For this review, take the finished solid that the model builds, in its own axes (mm). A direction names the side the tool comes from. Give positions to 0.01 mm unless a question says otherwise; leave off trailing zeros. Order: outer loops, then holes, each group sorted by start corner. A loop starts at its lowest first (then second) coordinate and runs counter-clockwise, first axis right, second up. Notation, with made-up numbers: (-11, -12) -> (-4, -12) arc R15 ccw to (-4, 11) -> close; hole circle Ø9 at (61.5, -27.75). An arc over 180 degrees is marked (long way). Use CSV: the item, a comma, the result in double quotes. Start each with the question number.
```python
from build123d import *

# Parameters (mm, degrees)
SKETCH_1_W               = 24
SKETCH_1_H               = 26
EXTRUDE_1_DEPTH          = 65
SKETCH_7_W               = 5
SKETCH_7_H               = 26
CUT_EXTRUDE_5_DEPTH      = 50
SKETCH_4_R               = 3
EXTRUDE_3_DEPTH          = 40
SKETCH_5_W               = 12.1
SKETCH_5_H               = 8
CUT_EXTRUDE_3_DEPTH      = 4
SKETCH_6_R               = 1
CUT_EXTRUDE_4_DEPTH      = 40
MIRROR_2_COPY_1_SKETCH_W = 5
MIRROR_2_COPY_1_SKETCH_H = 26
MIRROR_2_COPY_1_DEPTH    = 50
MIRROR_2_COPY_2_SKETCH_R = 3
MIRROR_2_COPY_2_DEPTH    = 40
MIRROR_2_COPY_3_SKETCH_W = 12.1
MIRROR_2_COPY_3_SKETCH_H = 8
MIRROR_2_COPY_3_DEPTH    = 4
MIRROR_2_COPY_4_SKETCH_R = 1
MIRROR_2_COPY_4_DEPTH    = 40
CUT_EXTRUDE_7_DEPTH      = 68.420693576
CUT_EXTRUDE_7_DEPTH_BACK = 68.420693576
CUT_EXTRUDE_8_REACH      = 83.979


with BuildPart() as part:
    # Эскиз1 → Бобышка-Вытянуть1 (new, symmetric)
    with BuildSketch(Plane.XY):
        with Locations((0, -0.287208972)):
            Rectangle(SKETCH_1_W, SKETCH_1_H)
    extrude(amount=EXTRUDE_1_DEPTH, both=True)

    # Эскиз7 → Вырез-Вытянуть5 (cut)
    with BuildSketch(Plane.XY.offset(65)):
        with Locations((-9.5, -0.287208972)):
            Rectangle(SKETCH_7_W, SKETCH_7_H)
    cut_extrude_5 = extrude(amount=-CUT_EXTRUDE_5_DEPTH, mode=Mode.SUBTRACT)

    # Эскиз4 → Бобышка-Вытянуть3 (add)
    with BuildSketch(Plane.XY.offset(65)):
        with BuildLine():
            ThreePointArc((-4, -10.287208972), (-4.878679656, -8.165888628), (-7, -7.287208972))
            Line((-7, -7.287208972), (-7, -13.287208972))
            ThreePointArc((-7, -13.287208972), (-4.878679656, -12.408529315), (-4, -10.287208972))
        make_face()
        with BuildLine():
            Line((-7, -13.287208972), (-7, -7.287208972))
            ThreePointArc((-7, -7.287208972), (-10, -10.287208972), (-7, -13.287208972))
        make_face()
        with Locations((-7, 9.712791028)):
            Circle(SKETCH_4_R)
    extrude_3 = extrude(amount=-EXTRUDE_3_DEPTH)

    # Эскиз5 → Вырез-Вытянуть3 (cut, symmetric)
    with BuildSketch(Plane.ZY.offset(7)):
        with Locations((45, -9.287208972)):
            Rectangle(SKETCH_5_W, SKETCH_5_H)
        with Locations((45, 8.712791028)):
            Rectangle(SKETCH_5_W, SKETCH_5_H)
    cut_extrude_3 = extrude(amount=CUT_EXTRUDE_3_DEPTH, both=True, mode=Mode.SUBTRACT)

    # Эскиз6 → Вырез-Вытянуть4 (cut)
    with BuildSketch(Plane.XY.offset(65)):
        with Locations((-7, 9.712791028)):
            Circle(SKETCH_6_R)
        with Locations((-7, -10.287208972)):
            Circle(SKETCH_6_R)
    cut_extrude_4 = extrude(amount=-CUT_EXTRUDE_4_DEPTH, mode=Mode.SUBTRACT)

    # Зеркальное отражение1: Вырез-Вытянуть5, Бобышка-Вытянуть3, Вырез-Вытянуть3, Вырез-Вытянуть4 across plane
    add(cut_extrude_5.mirror(Plane.XY), mode=Mode.SUBTRACT)
    add(extrude_3.mirror(Plane.XY))
    add(cut_extrude_3.mirror(Plane.XY), mode=Mode.SUBTRACT)
    add(cut_extrude_4.mirror(Plane.XY), mode=Mode.SUBTRACT)

    # Зеркальное отражение2: Вырез-Вытянуть5, Бобышка-Вытянуть3, Вырез-Вытянуть3, Вырез-Вытянуть4 across plane
    add(cut_extrude_5.mirror(Plane(origin=(0, 0, 0), x_dir=(0, 0, 1), z_dir=(1, 0, 0))), mode=Mode.SUBTRACT)
    add(extrude_3.mirror(Plane(origin=(0, 0, 0), x_dir=(0, 0, 1), z_dir=(1, 0, 0))))
    add(cut_extrude_3.mirror(Plane(origin=(0, 0, 0), x_dir=(0, 0, 1), z_dir=(1, 0, 0))), mode=Mode.SUBTRACT)
    add(cut_extrude_4.mirror(Plane(origin=(0, 0, 0), x_dir=(0, 0, 1), z_dir=(1, 0, 0))), mode=Mode.SUBTRACT)

    # Зеркальное отражение2 copy 1 sketch → Зеркальное отражение2 copy 1 (cut)
    with BuildSketch(Plane(origin=(0, 0, -65), x_dir=(-1, 0, 0), z_dir=(0, 0, -1))):
        with Locations((-9.5, -0.287208972)):
            Rectangle(MIRROR_2_COPY_1_SKETCH_W, MIRROR_2_COPY_1_SKETCH_H)
    extrude(amount=-MIRROR_2_COPY_1_DEPTH, mode=Mode.SUBTRACT)

    # Зеркальное отражение2 copy 2 sketch → Зеркальное отражение2 copy 2 (add)
    with BuildSketch(Plane(origin=(0, 0, -65), x_dir=(-1, 0, 0), z_dir=(0, 0, -1))):
        with BuildLine():
            ThreePointArc((-4, -10.287208972), (-4.878679656, -8.165888628), (-7, -7.287208972))
            Line((-7, -7.287208972), (-7, -13.287208972))
            ThreePointArc((-7, -13.287208972), (-4.878679656, -12.408529315), (-4, -10.287208972))
        make_face()
        with BuildLine():
            Line((-7, -13.287208972), (-7, -7.287208972))
            ThreePointArc((-7, -7.287208972), (-10, -10.287208972), (-7, -13.287208972))
        make_face()
        with Locations((-7, 9.712791028)):
            Circle(MIRROR_2_COPY_2_SKETCH_R)
    extrude(amount=-MIRROR_2_COPY_2_DEPTH)

    # Зеркальное отражение2 copy 3 sketch → Зеркальное отражение2 copy 3 (cut, symmetric)
    with BuildSketch(Plane(origin=(7, 0, 0), x_dir=(0, 0, -1), z_dir=(1, 0, 0))):
        with Locations((45, -9.287208972)):
            Rectangle(MIRROR_2_COPY_3_SKETCH_W, MIRROR_2_COPY_3_SKETCH_H)
        with Locations((45, 8.712791028)):
            Rectangle(MIRROR_2_COPY_3_SKETCH_W, MIRROR_2_COPY_3_SKETCH_H)
    extrude(amount=MIRROR_2_COPY_3_DEPTH, both=True, mode=Mode.SUBTRACT)

    # Зеркальное отражение2 copy 4 sketch → Зеркальное отражение2 copy 4 (cut)
    with BuildSketch(Plane(origin=(0, 0, -65), x_dir=(-1, 0, 0), z_dir=(0, 0, -1))):
        with Locations((-7, 9.712791028)):
            Circle(MIRROR_2_COPY_4_SKETCH_R)
        with Locations((-7, -10.287208972)):
            Circle(MIRROR_2_COPY_4_SKETCH_R)
    extrude(amount=-MIRROR_2_COPY_4_DEPTH, mode=Mode.SUBTRACT)

    # Эскиз9 → Вырез-Вытянуть7 (cut, two sides: drawn at the far end of the back side and taken through both)
    with BuildSketch(Plane.XY.offset(-CUT_EXTRUDE_7_DEPTH_BACK)):
        with BuildLine():
            Line((0, -9.287208972), (0, 8.712791028))
            Line((0, 8.712791028), (-2.101020514, 8.712791028))
            ThreePointArc((-2.101020514, 8.712791028), (-2.775255129, 7.038556414), (-4, 5.712791028))
            Line((-4, 5.712791028), (-4, -6.287208972))
            ThreePointArc((-4, -6.287208972), (-2.775255129, -7.612974358), (-2.101020514, -9.287208972))
            Line((-2.101020514, -9.287208972), (0, -9.287208972))
        make_face()
        with BuildLine():
            Line((2.101020514, 8.712791028), (0, 8.712791028))
            Line((0, 8.712791028), (0, -9.287208972))
            Line((0, -9.287208972), (2.101020514, -9.287208972))
            ThreePointArc((2.101020514, -9.287208972), (2.775255129, -7.612974358), (4, -6.287208972))
            Line((4, -6.287208972), (4, 5.712791028))
            ThreePointArc((4, 5.712791028), (2.775255129, 7.038556414), (2.101020514, 8.712791028))
        make_face()
    extrude(amount=CUT_EXTRUDE_7_DEPTH + CUT_EXTRUDE_7_DEPTH_BACK, mode=Mode.SUBTRACT)

    # Эскиз10 → Вырез-Вытянуть8 (cut, up to next)
    with BuildSketch(Plane.XY.offset(15), mode=Mode.PRIVATE) as cut_extrude_8_sk1:
        Polygon((-7, -13.287208972), (-12, -8.287208972), (-12, -13.287208972), align=None)
    cut_extrude_8_tool1 = extrude(cut_extrude_8_sk1.sketch, amount=-CUT_EXTRUDE_8_REACH, mode=Mode.PRIVATE) & part.part
    # Эскиз10 → Вырез-Вытянуть8 (cut, up to next)
    with BuildSketch(Plane.XY.offset(15), mode=Mode.PRIVATE) as cut_extrude_8_sk2:
        Polygon((7, -13.287208972), (12, -13.287208972), (12, -8.287208972), align=None)
    cut_extrude_8_tool2 = extrude(cut_extrude_8_sk2.sketch, amount=-CUT_EXTRUDE_8_REACH, mode=Mode.PRIVATE) & part.part
    add(cut_extrude_8_tool1.solids().sort_by_distance((-10.333333, -11.620542, 15))[0], mode=Mode.SUBTRACT)
    add(cut_extrude_8_tool2.solids().sort_by_distance((10.333333, -11.620542, 15))[0], mode=Mode.SUBTRACT)


solid = part.part
```
1. For faces 1 (the face through (-10, 9.8, -32.1)), 2 (the face through (6, -9, 38.95)), 3 (the face through (6, 4.713, -45)), 4 (the face through (2.762, -7.634, -0.91)), list the 3-axis set-ups (+Z, -Z, +X, -X, +Y, -Y) from which the entire face can be reached by the end or side of a thin tool; tool diameter is ignored.
2. Consider section A-A (y = 0.5). State the section outline as (x, z) points, plus the area to 3 significant figures.
3. To check wall thickness, follow L1, parallel to Z at x = -6.25, y = -8.5; L2, parallel to X at y = 4.25, z = 4; L3, parallel to X at y = -1, z = 50.5. State the ranges of each line that lie inside material, in increasing order. Write a range as [from, to].
4. Draft analysis for pull direction Y (two halves, no side actions). For faces 5 (the face through (3, -10, -45)), 6 (the face through (-10, -10.2, -58.1)), 7 (the face through (-5, -5.287, -45)), state which applies: +Y half, -Y half, draft (parallel to the pull), parting line (faces both ways), or undercut.
5. Consider section C-C (z = -32). State the section outline as (x, y) points.
6. Clearance check with flat-ended pins moving along their axes: P1, Ø13, axis at y = 3.5, z = 45, coming from the -X side; P2, Ø1.2, axis at x = -7, y = -10.29, coming from the +Z side; P3, Ø1, axis at y = 1, z = 31, coming from the +X side. State where each tip first meets the part, or that it passes through.
7. Consider section B-B (z = 7.5). State the section outline as (x, y) points.
Answer list:
1,face 1,"-Z, -X"
1,face 2,"+X, -Y"
1,face 3,"+X, -X, +Y"
1,face 4,"+Z, -Z"
2,outline,"(-12, -15) -> (-7, -15) -> (-7, -65) -> (-4, -65) -> (-4, 65) -> (-7, 65) -> (-7, 15) -> (-12, 15) -> close; (4, -65) -> (7, -65) -> (7, -15) -> (12, -15) -> (12, 15) -> (7, 15) -> (7, 65) -> (4, 65) -> close"
2,area,"1,080 mm2"
3,L1,"[-65, -51.05], [-38.95, 38.95], [51.05, 65]"
3,L2,"[-12, -4], [4, 12]"
3,L3,"[-7, -4], [4, 7]"
4,face 5,"draft"
4,face 6,"undercut"
4,face 7,"-Y half"
5,outline,"(-7, -13.29) -> (7, -13.29) arc R3 ccw to (7, -7.29) -> (7, 6.71) arc R3 ccw to (7, 12.71) -> (-7, 12.71) arc R3 ccw to (-7, 6.71) -> (-7, -7.29) arc R3 ccw to start; hole circle Ø2 at (-7, -10.29); hole circle Ø2 at (-7, 9.71); hole (-4, -6.29) arc R5 cw to (-2.1, -9.29) -> (2.1, -9.29) arc R5 cw to (4, -6.29) -> (4, 5.71) arc R5 cw to (2.1, 8.71) -> (-2.1, 8.71) arc R5 cw to (-4, 5.71) -> close; hole circle Ø2 at (7, -10.29); hole circle Ø2 at (7, 9.71)"
6,P1,"x = -7"
6,P2,"z = 25"
6,P3,"x = 7"
7,outline,"(-12, -8.29) -> (-7, -13.29) -> (7, -13.29) -> (12, -8.29) -> (12, 12.71) -> (-12, 12.71) -> close; hole (-4, -6.29) arc R5 cw to (-2.1, -9.29) -> (2.1, -9.29) arc R5 cw to (4, -6.29) -> (4, 5.71) arc R5 cw to (2.1, 8.71) -> (-2.1, 8.71) arc R5 cw to (-4, 5.71) -> close"
